Design review of the part built by this model. Coordinates are the model's own, in mm. Coordinates: 2 decimals unless noted, no trailing zeros. Write each loop counter-clockwise with the first axis right and the second up, starting at its lowest first coordinate (ties: lowest second). Pieces come first, ordered by that corner, then holes.
Q1. Add section C-C, the plane y = -14.5. Give the boundary of the cut face in (x, z), plus the area to 3 significant figures.
Q2. The part is to be moulded in two halves that separate along X. For faces 1 (the face through (-2.796, -10.14, 21.298)), 2 (the face through (-6.3, -19.88, 47.97)), 3 (the face through (21, -20, -10)), say which applies: +X half, -X half, draft (parallel to the pull), parting line (faces both ways), or undercut.
Q3. Add section A-A, the plane z = 0. Give the boundary of the cut face in (x, y), plus the area to 3 significant figures.
Q4. Add section B-B, the plane x = 0. Give the boundary of the cut face in (y, z), plus the area to 3 significant figures.
Q5. Clearance check with flat-ended pins moving along their axes: pin 1 Ø10 at (x, y) = (7.5, -16) entering from -Z; pin 2 Ø4 at (y, z) = (-13.5, -23.5) entering from -X; pin 3 Ø3 at (y, z) = (-7, 5) entering from -X. State where each tip first meets the part, or that it passes through.
Q6. To check wall thickness, follow probe 1 along Z at (x, y) = (0, -8.75); probe 2 along Z at (x, y) = (-11.5, -3.5); probe 3 along X at (y, z) = (-1.5, 4). State the ranges of each line that lie inside material, in increasing order.
from build123d import *

# Parameters (mm, degrees)
F0_R     = 50.8
F1_DEPTH = 20
F3_SIZE  = 2.54
F2_R     = 21.480833
F4_DEPTH = 20


with BuildPart() as f1:
    # F0 (on Front) → F1 (new body)
    with BuildSketch(Plane.XZ):
        Circle(F0_R)
    extrude(amount=F1_DEPTH)

    # F3
    f3_edges = [f1.edges().sort_by_distance(p)[0] for p in [
        (-50.8, -20, 0),
        (-50.8, 0, 0),
    ]]
    chamfer(f3_edges, length=F3_SIZE)

    # F2 (on face) → F4 (cut, through all)
    with BuildSketch(Plane.XZ.offset(20)):
        Circle(F2_R)
    extrude(amount=-F4_DEPTH, mode=Mode.SUBTRACT)


solid = f1.part
Here are the results:
1. outline: circle Ø101.6 at (0, 0); hole circle Ø42.96 at (0, 0)
1. area: 6,660 mm2
2. face 1: undercut
2. face 2: parting line
2. face 3: draft
3. outline: (-50.8, -17.46) - (-48.26, -20) - (-21.48, -20) - (-21.48, 0) - (-48.26, 0) - (-50.8, -2.54) - close; (21.48, -20) - (48.26, -20) - (50.8, -17.46) - (50.8, -2.54) - (48.26, 0) - (21.48, 0) - close
3. area: 1,160 mm2
4. outline: (-20, -48.26) - (-17.46, -50.8) - (-2.54, -50.8) - (0, -48.26) - (0, -21.48) - (-20, -21.48) - close; (-20, 21.48) - (0, 21.48) - (0, 48.26) - (-2.54, 50.8) - (-17.46, 50.8) - (-20, 48.26) - close
4. area: 1,160 mm2
5. pin 1: stops at z = -50.74
5. pin 2: stops at x = -46.03
5. pin 3: stops at x = -50.68
6. probe 1: z = -50.8 to -21.48, 21.48 to 50.8
6. probe 2: z = -49.48 to -18.14, 18.14 to 49.48
6. probe 3: x = -49.6 to -21.11, 21.11 to 49.6
